Geometry: final body of the model. Coordinates: model frame, mm. Face numbers are marked on the shaded views. A direction names the side the tool comes from. Round coordinates to 2 decimals unless told otherwise and drop trailing zeros. Order: outer loops, then holes, each group sorted by start corner. A loop starts at its lowest first (then second) coordinate and runs counter-clockwise, first axis right, second up. Notation, with made-up numbers: (17, 37) -> (62, 37) arc R28 ccw to (62, 63) -> close; hole circle Ø3 at (-16, 4.25). An arc over 180 degrees is marked (long way). Put each result on its own line as item: value.
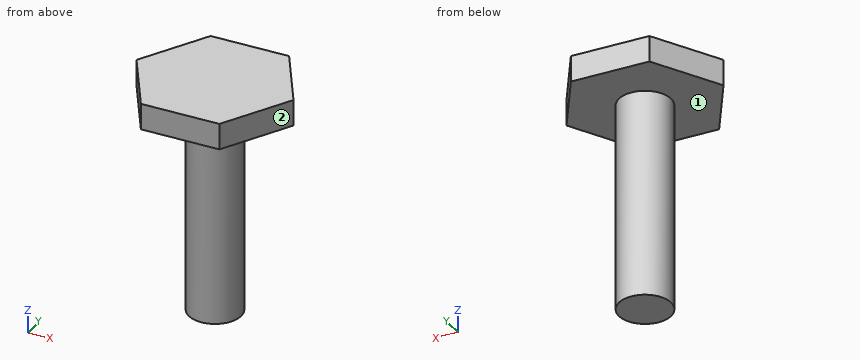
```python
from build123d import *

# Parameters (mm, degrees)
SKETCH1_R           = 3.175
BOSS_EXTRUDE1_DEPTH = 12.7
BOSS_EXTRUDE3_DEPTH = 3.175


with BuildPart() as part:
    # Sketch1 → Boss-Extrude1 (new, symmetric)
    with BuildSketch(Plane.XY):
        Circle(SKETCH1_R)
    extrude(amount=BOSS_EXTRUDE1_DEPTH, both=True)

    # Sketch2 → Boss-Extrude3 (add)
    with BuildSketch(Plane.XY.offset(12.7)):
        Polygon((9.525, 0), (4.7625, 8.248891971), (-4.7625, 8.248891971), (-9.525, 0), (-4.7625, -8.248891971), (4.7625, -8.248891971), align=None)
    extrude(amount=BOSS_EXTRUDE3_DEPTH)


solid = part.part
```
1. Material intervals for probe 1 along Z at (x, y) = (3.5, -2.75) (3 decimals); probe 2 along X at (y, z) = (0.5, 9.75); probe 3 along Y at (x, z) = (1.75, 2.5), sorted ascending.
Ans:
probe 1: 12.7 to 15.875
probe 2: -3.14 to 3.14
probe 3: -2.65 to 2.65
2. Contact query for flat-ended pins moving along their axis: P1, Ø6, axis at x = -3, z = -6.5, coming from the +Y side (3 decimals); P2, Ø1, axis at x = -3.5, y = -5.5, coming from the -Z side; P3, Ø3, axis at y = 3, z = -6, coming from the -X side. Output: stop coordinate, or through.
Ans:
P1: y = 3.175
P2: z = 12.7
P3: x = -2.8
3. Set-up query: the marked faces 1 and 2. Return all of +Z, -Z, +X, -X, +Y, -Y with unobstructed straight access to the full face (end or side cutting, diameter ignored); none if empty.
Ans:
face 1: -Z
face 2: +Z, -Z, +X, -Y
4. Cut plane A-A on x = 0. Return loops of the section in (y, z) (3 decimals).
Ans:
outline: (-8.249, 12.7) -> (-3.175, 12.7) -> (-3.175, -12.7) -> (3.175, -12.7) -> (3.175, 12.7) -> (8.249, 12.7) -> (8.249, 15.875) -> (-8.249, 15.875) -> close
5. Cut plane C-C on y = -1. Return loops of the section in (x, z) (3 decimals).
Ans:
outline: (-8.948, 12.7) -> (-3.013, 12.7) -> (-3.013, -12.7) -> (3.013, -12.7) -> (3.013, 12.7) -> (8.948, 12.7) -> (8.948, 15.875) -> (-8.948, 15.875) -> close
6. Cut plane B-B on z = 9.75. Return loops of the section in (x, y) (3 decimals), and give its area (3 significant figures).
Ans:
outline: circle Ø6.35 at (0, 0)
area: 31.7 mm²
7. Cut plane D-D on y = -6.5. Return loops of the section in (x, z) (3 decimals).
Ans:
outline: (-5.772, 12.7) -> (5.772, 12.7) -> (5.772, 15.875) -> (-5.772, 15.875) -> close
